from build123d import *

# Parameters (mm, degrees)
F0_R     = 6.425
F1_DEPTH = 12
F2_R     = 1.5
F3_DEPTH = 12.5
F5_DEPTH = 3.25
F6_W     = 3.25
F6_H     = 1.2716361485
F6_W_2   = 2.4
F6_H_2   = 1.6
F6_H_3   = 3
F6_H_4   = 1.8378814235
F7_DEPTH = 12.5
F8_R     = 1.25
F9_DEPTH = 4.5


with BuildPart() as f1:
    # F0 (on Top) → F1 (new body)
    with BuildSketch(Plane.XY):
        Circle(F0_R)
    extrude(amount=-F1_DEPTH)

    # F2 (on Front) → F3 (cut, symmetric)
    with BuildSketch(Plane.XZ):
        with Locations((0, -8.6621185765)):
            Circle(F2_R)
    extrude(amount=F3_DEPTH, both=True, mode=Mode.SUBTRACT)

    # F4 (on Front) → F5 (cut)
    with BuildSketch(Plane.XZ):
        with BuildLine():
            Line((6.425, -12), (2.7726078369, -6.7377301586))
            ThreePointArc((2.7726078369, -6.7377301586), (0, -5.2871185765), (-2.7726078369, -6.7377301586))
            Line((-2.7726078369, -6.7377301586), (-6.425, -12))
            Line((-6.425, -12), (6.425, -12))
        make_face()
    extrude(amount=-F5_DEPTH, mode=Mode.SUBTRACT)

    # F6 (on Right) → F7 (cut, symmetric)
    with BuildSketch(Plane.YZ):
        with Locations((1.625, -11.3641819257)):
            Rectangle(F6_W, F6_H)
        with Locations((-5.225, -6.3621185765)):
            Rectangle(F6_W_2, F6_H_2)
        with Locations((-5.225, -8.6621185765)):
            Rectangle(F6_W_2, F6_H_3)
        with Locations((-5.225, -11.0810592882)):
            Rectangle(F6_W_2, F6_H_4)
    extrude(amount=F7_DEPTH, both=True, mode=Mode.SUBTRACT)

    # F8 (on face) → F9 (join)
    with BuildSketch(Plane.XY):
        Circle(F8_R)
    extrude(amount=F9_DEPTH)


solid = f1.part
Here's how the part is built. I have some questions about the finished solid (model axes, mm). A direction names the side the tool comes from. Round coordinates to 2 decimals unless told otherwise and drop trailing zeros. Loops run counter-clockwise (first coordinate to the right, second up) from the corner with the lowest first, then second, coordinate; pieces in that order, holes last. Notation, with made-up numbers: (6, 37.5) - (41, 37.5) arc R7 ccw to (41, 44.5) - close; hole circle Ø10 at (-14, 61). An arc over 180 degrees is marked (long way). One line per question, with ' | ' between items. Start each with the question number.
Q1. I want a section at D-D (x = -5.25). Write out the boundary of the cut face in (y, z), then the cut area to 3 significant figures.
Q2. Will these pins go through, and if not, where does the flat tip stop? pin 1 (3.5 mm diameter, centred on x = 0.5, z = -7.5, fed in from -Y) (3 decimals); pin 2 (4 mm diameter, centred on x = -4, z = -5, fed in from +Y); pin 3 (1.9 mm diameter, centred on x = -1.5, y = -6, fed in from -Z).
Q3. For faces 1 (the flat face through (0, 5, -12)), 2 (the flat face through (1, -4.025, -10)), 3 (the flat face through (6, 1, -10.728)), 4 (the cylindrical face through (0.046, 1.602, -5.287)), which set-ups out of +Z, -Z, +X, -X, +Y, -Y let a thin tool reach every point of the face, with its end or its side?
Q4. I want a section at C-C (y = -2). Write out the boundary of the cut face in (x, z).
Q5. Please list where these lines run through material, in increasing order: line 1 (Z direction, x = 0, y = 4.15); line 2 (Z direction, x = 0, y = -0.8); line 3 (Y direction, x = 3.25, z = -8) (3 decimals). Write a range as [from, to].
Q6. I want a section at A-A (x = 0). Write out the boundary of the cut face in (y, z) (3 decimals).
Q7. We'd pull the mould along X, two halves only. Please class faces 5 (the flat face through (1, 3.25, -10)), 6 (the cylindrical face through (-0.325, 4.818, -10.126)), 7 (the cylindrical face through (-0.27, -1.22, 2.22)), 8 (the flat face through (0, -2, -12)): +X half, -X half, draft (parallel to the pull), parting line (faces both ways), or undercut.
Q8. I want a section at B-B (z = -8). Write out the boundary of the cut face in (x, y) (3 decimals), then the cut area to 3 significant figures.
Response values:
1) outline: (-3.7, -12) - (0, -12) - (0, -10.31) - (3.25, -10.31) - (3.25, -12) - (3.7, -12) - (3.7, 0) - (-3.7, 0) - close | area: 83.4 mm²
2) pin 1: stops at y = -4.025 | pin 2: stops at y = 6.11 | pin 3: stops at z = -5.56
3) face 1: -Z, +X, -X, +Y, -Y | face 2: -Z, +X, -X, -Y | face 3: -Z, +X, -X, +Y | face 4: -Z
4) outline: (-6.11, -12) - (6.11, -12) - (6.11, 0) - (-6.11, 0) - close; hole circle Ø3 at (0, -8.66)
5) line 1: z = [-12, -10.16], [-7.16, 0] | line 2: z = [-12, -10.16], [-7.16, 4.5] | line 3: y = [-4.025, 0], [3.25, 5.542]
6) outline: (-6.425, -5.562) - (-4.025, -5.562) - (-4.025, -7.162) - (0, -7.162) - (0, -5.287) - (3.25, -5.287) - (3.25, -7.162) - (6.425, -7.162) - (6.425, 0) - (1.25, 0) - (1.25, 4.5) - (-1.25, 4.5) - (-1.25, 0) - (-6.425, 0) - close; (-4.025, -12) - (0, -12) - (0, -10.162) - (-4.025, -10.162) - close; (3.25, -12) - (6.425, -12) - (6.425, -10.162) - (3.25, -10.162) - close
7) face 5: undercut | face 6: undercut | face 7: parting line | face 8: draft
8) outline: (-5.008, -4.025) - (-1.346, -4.025) - (-1.346, 0) - (-3.649, 0) - (-3.649, 3.25) - (-1.346, 3.25) - (-1.346, 6.282) arc R6.425 ccw to start; (1.346, -4.025) - (5.008, -4.025) arc R6.425 ccw to (1.346, 6.282) - (1.346, 3.25) - (3.649, 3.25) - (3.649, 0) - (1.346, 0) - close | area: 70.0 mm²
